Here's the drawing with two shaded views (mm, measured from the low corner). I have some questions. A direction names the side the tool comes from. Give positions to 0.01 mm unless a question says otherwise; leave off trailing zeros. Loops run counter-clockwise (first coordinate to the right, second up) from the corner with the lowest first, then second, coordinate; pieces in that order, holes last. Notation, with made-up numbers: (89.5, 71) - (118.5, 71) arc R15 ccw to (118.5, 93) - close; hole circle Ø1 at (44, -23.5). An arc over 180 degrees is marked (long way). Use one line per item in the form item = value.
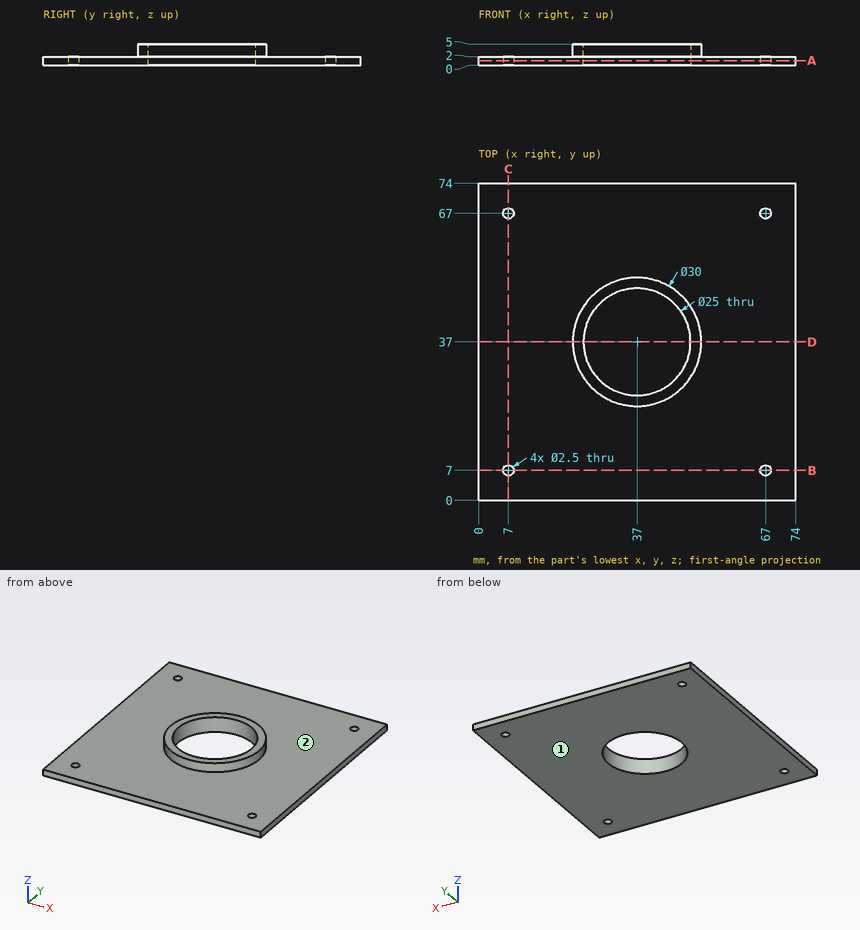
(1) For P1, Ø12, axis at x = 14.5, y = 36, coming from the +Z side; P2, Ø1.5, axis at x = 67, y = 67, coming from the +Z side, each with a flat end and sliding along its axis, tell me the tip position at first contact or that it passes through.
Geometry says:
P1 = 2
P2 = through
(2) If we section it at D-D (y = 37): List the corners of the cut face in (x, z) for me.
Geometry says:
outline = (0, 0) - (24.5, 0) - (24.5, 5) - (22, 5) - (22, 2) - (0, 2) - close; (49.5, 0) - (74, 0) - (74, 2) - (52, 2) - (52, 5) - (49.5, 5) - close
(3) For the marked faces 1 and 2, which set-ups out of +Z, -Z, +X, -X, +Y, -Y let a thin tool reach every point of the face, with its end or its side?
Geometry says:
face_1 = -Z, +X, -X, +Y, -Y
face_2 = +Z
(4) If I drill on probe 1 along Y at (x, z) = (67, 1.55); probe 2 along Z at (x, y) = (32, 69.5), over which ranges is the centre line in solid material (lowest first)?
Geometry says:
probe_1 = 0 to 5.75, 8.25 to 65.75, 68.25 to 74
probe_2 = 0 to 2
(5) If we section it at A-A (z = 1.1): List the corners of the cut face in (x, y) for me, plus the area to 3 significant figures.
Geometry says:
outline = (0, 0) - (74, 0) - (74, 74) - (0, 74) - close; hole circle Ø2.5 at (7, 7); hole circle Ø2.5 at (7, 67); hole circle Ø25 at (37, 37); hole circle Ø2.5 at (67, 7); hole circle Ø2.5 at (67, 67)
area = 4,970 mm²
(6) If we section it at B-B (y = 7): List the corners of the cut face in (x, z) for me, plus the area to 3 significant figures.
Geometry says:
outline = (0, 0) - (5.75, 0) - (5.75, 2) - (0, 2) - close; (8.25, 0) - (65.75, 0) - (65.75, 2) - (8.25, 2) - close; (68.25, 0) - (74, 0) - (74, 2) - (68.25, 2) - close
area = 138 mm²
